Part print with two shaded views. Sizes in mm from the minimum x, y, z corner. Round coordinates to 2 decimals unless told otherwise and drop trailing zeros. Loops run counter-clockwise (first coordinate to the right, second up) from the corner with the lowest first, then second, coordinate; pieces in that order, holes last. Notation, with made-up numbers: (-1.75, 46.5) -> (11.25, 46.5) arc R24 ccw to (11.25, 71.5) -> close; hole circle Ø10 at (52, 24.5). An arc over 180 degrees is marked (long way). Use a Markdown table: item, result. Add a question column.
Item 1: Cut at D-D, the plane z = 5. List the corners of the cut face in (x, y), plus the area to 3 significant figures.
Item 2: Cut at A-A, the plane y = 0.7. List the corners of the cut face in (x, z), plus the area to 3 significant figures.
Item 3: Probe line 1 (Z direction, x = 2.3, y = 0.8); line 2 (X direction, y = 0.45, z = 4.75); line 3 (Y direction, x = 2.15, z = 5.75). List the from-to ranges inside material, lowest first. Write a range as [from, to].
Item 4: Cut at C-C, the plane y = 0.2. List the corners of the cut face in (x, z).
Item 5: Cut at B-B, the plane x = 3.4. List the corners of the cut face in (y, z), plus the area to 3 significant figures.
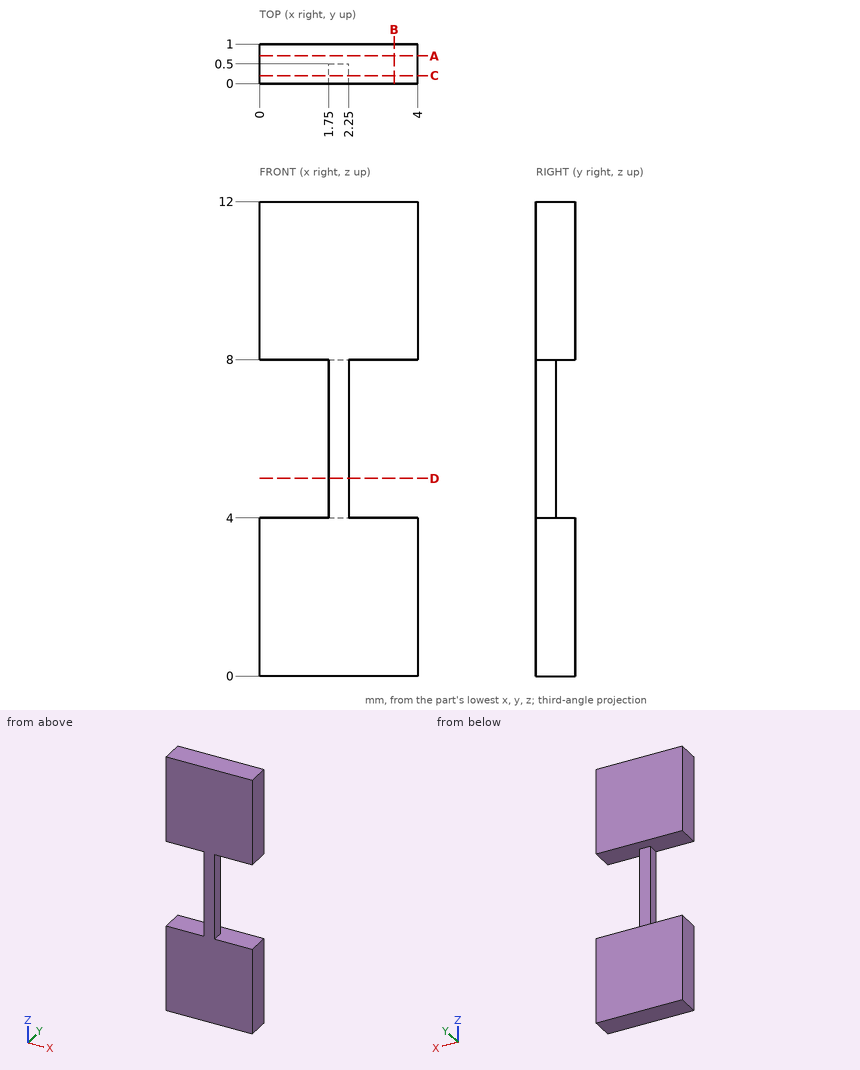
A:
| question | item | result |
|---|---|---|
| 1 | outline | (1.75, 0) -> (2.25, 0) -> (2.25, 0.5) -> (1.75, 0.5) -> close |
| 1 | area | 0.250 mm^2 |
| 2 | outline | (0, 0) -> (4, 0) -> (4, 4) -> (0, 4) -> close; (0, 8) -> (4, 8) -> (4, 12) -> (0, 12) -> close |
| 2 | area | 32.0 mm^2 |
| 3 | line 1 | z = [0, 4], [8, 12] |
| 3 | line 2 | x = [1.75, 2.25] |
| 3 | line 3 | y = [0, 0.5] |
| 4 | outline | (0, 0) -> (4, 0) -> (4, 4) -> (2.25, 4) -> (2.25, 8) -> (4, 8) -> (4, 12) -> (0, 12) -> (0, 8) -> (1.75, 8) -> (1.75, 4) -> (0, 4) -> close |
| 5 | outline | (0, 0) -> (1, 0) -> (1, 4) -> (0, 4) -> close; (0, 8) -> (1, 8) -> (1, 12) -> (0, 12) -> close |
| 5 | area | 8.00 mm^2 |
